For this review, take the finished solid that the model builds, in its own axes (mm). Coordinates: 2 decimals unless noted, no trailing zeros. Order: outer loops, then holes, each group sorted by start corner. A loop starts at its lowest first (then second) coordinate and runs counter-clockwise, first axis right, second up. Notation, with made-up numbers: (-10.75, 26.5) -> (15.25, 26.5) arc R24 ccw to (15.25, 65.5) -> close; hole circle Ø3 at (69, 88). An arc over 180 degrees is marked (long way). Return JSON: item names as keys, results as strings. Group by question number.
Item 1: Take a section at A-A (x = 3). Write out the cut boundary in (y, z) (3 decimals).
Item 2: Take a section at B-B (x = 21.5). Write out the cut boundary in (y, z) (3 decimals), then the cut area to 3 significant figures.
Item 3: For line 1 along Y through (x, z) = (-27, 2.65) (3 decimals); line 2 along X through (y, z) = (-42, 1.85) (3 decimals); line 3 along Y through (x, z) = (-25, 3) (3 decimals), list the stretches that pass through material, from the lowest coordinate up.
Item 4: Take a section at C-C (z = 1.45). Count the separate pieces of the cut face and the enclosed holes in it, then the cut area to 3 significant figures.
Item 5: Insertion check: pin 1 (3.5 mm diameter, centred on x = 57.15, y = -88.9, fed in from +Z) (3 decimals). The pin has a flat end and moves straight along its axis. Give the tip position at first contact, or say it passes through.
```python
from build123d import *

# Parameters (mm, degrees)
PAD_DEPTH       = 3.175
SKETCH001_R     = 1.5
POCKET_DEPTH    = 3.176
POCKET001_DEPTH = 3.176
SKETCH003_R     = 1.5
POCKET002_DEPTH = 5
POCKET003_DEPTH = 3.176
SKETCH005_R     = 1.5
POCKET004_DEPTH = 3.176
SKETCH006_R     = 1.5
POCKET005_DEPTH = 3.176


with BuildPart() as part:
    # Sketch → Pad (new body)
    with BuildSketch(Plane.XY):
        with BuildLine():
            ThreePointArc((-57.785, 92.075), (-59.581051, 91.331051), (-60.325, 89.535))
            Line((-60.325, -89.535), (-60.325, 89.535))
            ThreePointArc((-60.325, -89.535), (-59.581051, -91.331051), (-57.785, -92.075))
            Line((57.785, -92.075), (-57.785, -92.075))
            ThreePointArc((57.785, -92.075), (59.581051, -91.331051), (60.325, -89.535))
            Line((60.325, 89.535), (60.325, -89.535))
            ThreePointArc((60.325, 89.535), (59.581051, 91.331051), (57.785, 92.075))
            Line((-57.785, 92.075), (57.785, 92.075))
        make_face()
    extrude(amount=PAD_DEPTH)

    # Sketch001 (on DatumPlane) → Pocket (cut, through all)
    with BuildSketch(Plane.XY.offset(3.175)):
        with Locations((-57.15, 88.9)):
            Circle(SKETCH001_R)
        with Locations((57.15, 88.9)):
            Circle(SKETCH001_R)
        with Locations((-57.15, -88.9)):
            Circle(SKETCH001_R)
        with Locations((57.15, -88.9)):
            Circle(SKETCH001_R)
        with Locations((-57.15, 0)):
            Circle(SKETCH001_R)
        with Locations((57.15, 0)):
            Circle(SKETCH001_R)
    extrude(amount=-POCKET_DEPTH, mode=Mode.SUBTRACT)

    # Sketch002 (on DatumPlane) → Pocket001 (cut, through all)
    with BuildSketch(Plane.XY.offset(3.175)):
        with BuildLine():
            ThreePointArc((-28.575, 81.28), (-29.473026, 80.908026), (-29.845, 80.01))
            Line((-29.845, 77.47), (-29.845, 80.01))
            ThreePointArc((-29.845, 77.47), (-29.473026, 76.571974), (-28.575, 76.2))
            Line((28.575, 76.2), (-28.575, 76.2))
            ThreePointArc((28.575, 76.2), (29.473026, 76.571974), (29.845, 77.47))
            Line((29.845, 80.01), (29.845, 77.47))
            ThreePointArc((29.845, 80.01), (29.473026, 80.908026), (28.575, 81.28))
            Line((-28.575, 81.28), (28.575, 81.28))
        make_face()
        with BuildLine():
            ThreePointArc((-28.575, 35.56), (-29.473026, 35.188026), (-29.845, 34.29))
            Line((-29.845, 31.75), (-29.845, 34.29))
            ThreePointArc((-29.845, 31.75), (-29.473026, 30.851974), (-28.575, 30.48))
            Line((28.575, 30.48), (-28.575, 30.48))
            ThreePointArc((28.575, 30.48), (29.473026, 30.851974), (29.845, 31.75))
            Line((29.845, 34.29), (29.845, 31.75))
            ThreePointArc((29.845, 34.29), (29.473026, 35.188026), (28.575, 35.56))
            Line((-28.575, 35.56), (28.575, 35.56))
        make_face()
    extrude(amount=-POCKET001_DEPTH, mode=Mode.SUBTRACT)

    # Sketch003 (on DatumPlane) → Pocket002 (cut)
    with BuildSketch(Plane.XY.offset(3.175)):
        with Locations((11.43, -8.89)):
            Circle(SKETCH003_R)
        with Locations((39.37, -8.89)):
            Circle(SKETCH003_R)
        with Locations((11.43, -41.91)):
            Circle(SKETCH003_R)
        with Locations((39.37, -41.91)):
            Circle(SKETCH003_R)
    extrude(amount=-POCKET002_DEPTH, mode=Mode.SUBTRACT)

    # Sketch004 (on DatumPlane) → Pocket003 (cut, through all)
    with BuildSketch(Plane.XY.offset(3.175)):
        with BuildLine():
            Line((13.97, -92.075), (13.97, -81.915))
            ThreePointArc((16.51, -79.375), (14.713949, -80.118949), (13.97, -81.915))
            Line((16.51, -79.375), (49.53, -79.375))
            ThreePointArc((52.07, -81.915), (51.326051, -80.118949), (49.53, -79.375))
            Line((52.07, -81.915), (52.07, -92.075))
            Line((52.07, -92.075), (52.07, -95.885))
            ThreePointArc((49.53, -98.425), (51.326051, -97.681051), (52.07, -95.885))
            Line((49.53, -98.425), (16.51, -98.425))
            ThreePointArc((13.97, -95.885), (14.713949, -97.681051), (16.51, -98.425))
            Line((13.97, -95.885), (13.97, -92.075))
        make_face()
    extrude(amount=-POCKET003_DEPTH, mode=Mode.SUBTRACT)

    # Sketch005 (on DatumPlane) → Pocket004 (cut, through all)
    with BuildSketch(Plane.XY.offset(3.175)):
        with Locations((-40.3225, 3.81)):
            Circle(SKETCH005_R)
        with Locations((-20.0025, 3.81)):
            Circle(SKETCH005_R)
        with Locations((-40.3225, -16.51)):
            Circle(SKETCH005_R)
        with Locations((-20.0025, -16.51)):
            Circle(SKETCH005_R)
    extrude(amount=-POCKET004_DEPTH, mode=Mode.SUBTRACT)

    # Sketch006 (on DatumPlane) → Pocket005 (cut, through all)
    with BuildSketch(Plane.XY.offset(3.175)):
        with Locations((-36.5125, -46.99)):
            Circle(SKETCH006_R)
        with Locations((-23.8125, -46.99)):
            Circle(SKETCH006_R)
        with Locations((-36.5125, -67.31)):
            Circle(SKETCH006_R)
        with Locations((-23.8125, -67.31)):
            Circle(SKETCH006_R)
    extrude(amount=-POCKET005_DEPTH, mode=Mode.SUBTRACT)


solid = part.part
```
Findings below:
{
 "1": {"outline": "(-92.075, 0) -> (30.48, 0) -> (30.48, 3.175) -> (-92.075, 3.175) -> close; (35.56, 0) -> (76.2, 0) -> (76.2, 3.175) -> (35.56, 3.175) -> close; (81.28, 0) -> (92.075, 0) -> (92.075, 3.175) -> (81.28, 3.175) -> close"},
 "2": {"outline": "(-79.375, 0) -> (30.48, 0) -> (30.48, 3.175) -> (-79.375, 3.175) -> close; (35.56, 0) -> (76.2, 0) -> (76.2, 3.175) -> (35.56, 3.175) -> close; (81.28, 0) -> (92.075, 0) -> (92.075, 3.175) -> (81.28, 3.175) -> close", "area": "512 mm2"},
 "3": {"line 1": "y = -92.075 to 30.48, 35.56 to 76.2, 81.28 to 92.075", "line 2": "x = -60.325 to 9.933, 12.927 to 37.873, 40.867 to 60.325", "line 3": "y = -92.075 to -68.226, -66.394 to -47.906, -46.074 to 30.48, 35.56 to 76.2, 81.28 to 92.075"},
 "4": {"separate pieces": "1", "enclosed holes": "20", "area": "21,000 mm2"},
 "5": {"pin 1": "stops at z = 3.175"}
}
